Autodesk Inventor part; units mm, degrees
ref_plane "YZ Plane" through (0, 0, 0) normal (1, 0, 0) x (0, 1, 0)
ref_plane "XZ Plane" through (0, 0, 0) normal (0, 1, 0) x (-1, 0, 0)
ref_plane "XY Plane" through (0, 0, 0) normal (0, 0, 1) x (1, 0, 0)
sketch "スケッチ1" plane through (0, 0, 0) normal (1, 0, 0) x (0, 1, 0)
  line L0 (0, 0) -> (105, 0)
  line L1 (105, 0) -> (31.5, 415)
  line L2 (31.5, 415) -> (0, 415)
  line L3 (0, 415) -> (0, 0)
  dimension "d0" = 415
  dimension "d1" = 31.5
  dimension "d2" = 105
revolve "回転1" add sketch "スケッチ1" angle 360 about axis through (0, 0, 415) along (0, 0, -1)
sketch "スケッチ2" plane through (0, 0, 0) normal (0, 0, -1) x (-1, 0, 0)
  line L0 (-137.5, -137.5) -> (137.5, -137.5)
  line L1 (137.5, -137.5) -> (137.5, 137.5)
  line L2 (137.5, 137.5) -> (-137.5, 137.5)
  line L3 (-137.5, 137.5) -> (-137.5, -137.5)
  line L4 (-137.5, -137.5) -> (137.5, 137.5) construction
  line L5 (137.5, -137.5) -> (-137.5, 137.5) construction
  point P0 (0, 0)
  dimension "d4" = 275
  dimension "d5" = 275
extrude "押し出し1" add sketch "スケッチ2" along normal blind 35
chamfer "面取り3" distance 35 distance2 25 1 edges at (0, 137.5, 0) measured on face at (-45.8333, 137.5, -11.6667)
chamfer "面取り4" distance 35 distance2 25 1 edges at (137.5, -12.5, 0) measured on face at (137.5, 37.5, -23.3333)
chamfer "面取り5" distance 35 distance2 25 1 edges at (-12.5, -137.5, 0) measured on face at (37.5, -137.5, -23.3333)
chamfer "面取り6" distance 35 distance2 25 1 edges at (-137.5, 0, 0) measured on face at (-137.5, -37.5, -23.3333)
shell "シェル1" thickness 11.5 removed faces 2 at (9.3296, 8.757, 415) at (45.8333, -45.8333, -35)
fillet "フィレット2" radius 5 19 edges at (0, -31.5, 415) (112.5001, 0, 0) (0, -112.5001, 0) (125, -125.0001, -17.5) (0, -105, 0) (125.0001, 125, -17.5) (0, 112.5001, 0) (-112.5001, 0, 0) (-125.0001, 125, -17.4999) (-125.0001, -125, -17.5) (0, -95.3578, -11.5) (0, -106.582, -11.5) (-106.582, 0, -11.5) (-114.9748, -114.9748, -23.25) (0, 106.582, -11.5) (106.582, 0, -11.5) (114.9748, 114.9748, -23.25) (-114.9748, 114.9748, -23.25) (114.9748, -114.9748, -23.25)
equation "\"d5\" = d4"
properties part number "mini_corn"
Part model, mm, in its own coordinate system. A direction names the side the tool comes from. Coordinates: 2 decimals unless noted, no trailing zeros. Use a Markdown table: item, result.
(1) Flat gauge pins, fed straight in: pin 1 (1.5 mm diameter, centred on x = -10, z = 16.5, fed in from -Y); pin 2 (5 mm diameter, centred on x = -50.5, y = -97.5, fed in from +Z); pin 3 (4 mm diameter, centred on y = 35, z = 244.5, fed in from +X). Where does each tip first touch, or does it go through?
A:
| item | result |
|---|---|
| pin 1 | stops at y = -101.74 |
| pin 2 | stops at z = 0.37 |
| pin 3 | stops at x = 52.2 |
(2) Probe L1, parallel to Z at x = 89, y = 74; L2, parallel to X at y = -33, z = 47.5; L3, parallel to X at y = 9, z = -17. List the from-to ranges inside material, lowest first.
A:
| item | result |
|---|---|
| L1 | z = -11.5 to 0 |
| L2 | x = -90.78 to -78.23, 78.23 to 90.78 |
| L3 | x = -124.64 to -110.51, 110.51 to 124.64 |
(3) Tool access for faces 1 (the cylindrical face through (-114.453, -114.514, -24.129)), 2 (the cylindrical face through (124.536, 124.596, -18.459)): list every direction of +Z, -Z, +X, -X, +Y, -Y with a clear straight run to the whole face (end or side of a thin tool).
A:
| item | result |
|---|---|
| face 1 | -Z |
| face 2 | +Z, +X, +Y |
(4) Pull direction X, two halves, no side cores. Call faces 3 (the cylindrical face through (-124.536, -124.596, -18.459)), 4 (the flat face through (14.3, 14, 415)), 5 (the flat face through (-115.62, 1.67, -24.15)): released by +X, released by -X, zero draft, split by the parting line, or undercut.
A:
| item | result |
|---|---|
| face 3 | released by -X |
| face 4 | zero draft |
| face 5 | undercut |
